Answer from the drawing. Dimensions are ordinates in mm from the lowest x, y and z of the part. Coordinates: 2 decimals unless noted, no trailing zeros. Loops run counter-clockwise (first coordinate to the right, second up) from the corner with the lowest first, then second, coordinate; pieces in that order, holes last. Notation, with made-up numbers: (7, -30.5) -> (65, -30.5) arc R24 cw to (65, -12.5) -> close; hole circle Ø10 at (-30.75, -9.75). An arc over 180 degrees is marked (long way). Use a Markdown table: item, result.
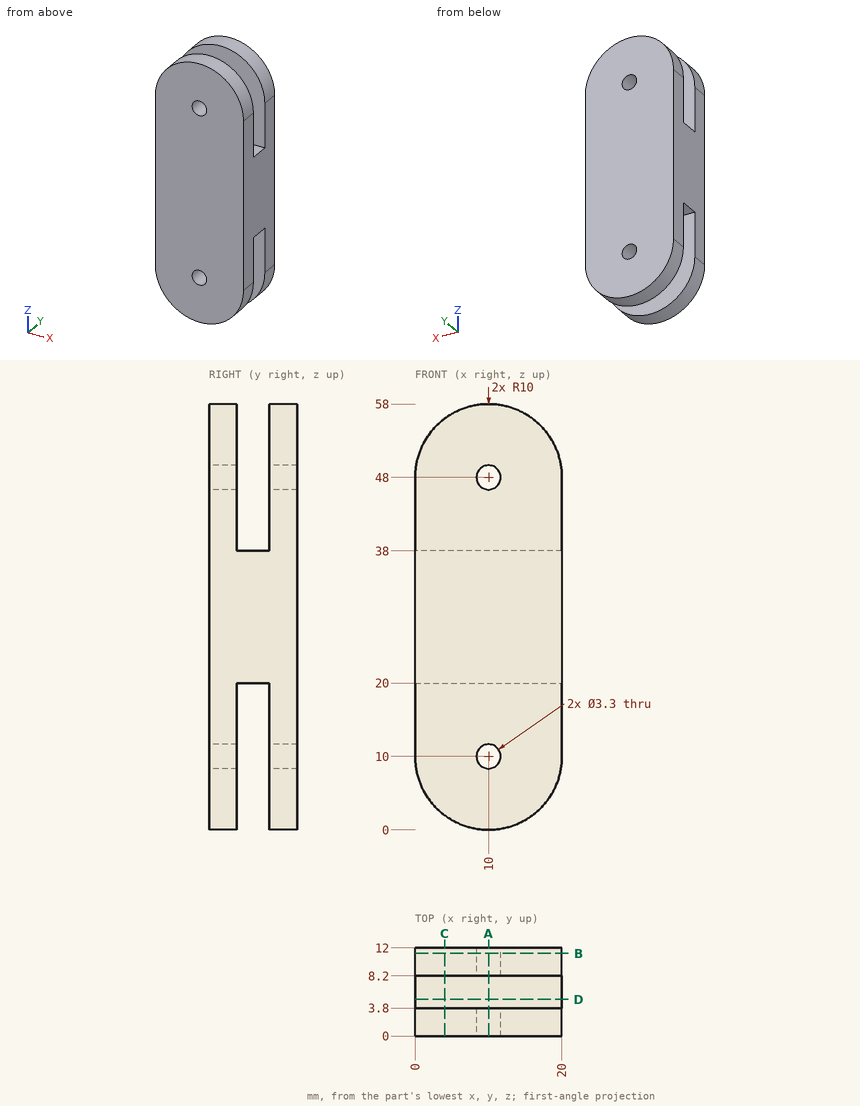
Q1. Consider line 1 (Z direction, x = 10, y = 10.1); line 2 (Y direction, x = 6, z = 8.5); line 3 (X direction, y = 9, z = 9). Determine where each line is inside the solid, lowest interval first. Write a range as [from, to].
Solved:
| item | result |
|---|---|
| line 1 | [0, 8.35], [11.65, 46.35], [49.65, 58] |
| line 2 | [0, 3.8], [8.2, 12] |
| line 3 | [0.05, 8.69], [11.31, 19.95] |
Q2. Section C-C on x = 4 is taken. Determine the outline of the cut face in (y, z).
Solved:
| item | result |
|---|---|
| outline | (0, 2) -> (3.8, 2) -> (3.8, 20) -> (8.2, 20) -> (8.2, 2) -> (12, 2) -> (12, 56) -> (8.2, 56) -> (8.2, 38) -> (3.8, 38) -> (3.8, 56) -> (0, 56) -> close |
Q3. Section B-B on y = 11.25 is taken. Determine the outline of the cut face in (x, z).
Solved:
| item | result |
|---|---|
| outline | (0, 10) arc R10 ccw to (20, 10) -> (20, 48) arc R10 ccw to (0, 48) -> close; hole circle Ø3.3 at (10, 10); hole circle Ø3.3 at (10, 48) |
Q4. Section A-A on x = 10 is taken. Determine the outline of the cut face in (y, z), and give its area (3 significant figures).
Solved:
| item | result |
|---|---|
| outline | (0, 0) -> (3.8, 0) -> (3.8, 8.35) -> (0, 8.35) -> close; (0, 11.65) -> (3.8, 11.65) -> (3.8, 20) -> (8.2, 20) -> (8.2, 11.65) -> (12, 11.65) -> (12, 46.35) -> (8.2, 46.35) -> (8.2, 38) -> (3.8, 38) -> (3.8, 46.35) -> (0, 46.35) -> close; (0, 49.65) -> (3.8, 49.65) -> (3.8, 58) -> (0, 58) -> close; (8.2, 0) -> (12, 0) -> (12, 8.35) -> (8.2, 8.35) -> close; (8.2, 49.65) -> (12, 49.65) -> (12, 58) -> (8.2, 58) -> close |
| area | 470 mm² |
Q5. Given pin 1 Ø3.5 at (x, y) = (10.5, 6) entering from +Z; pin 2 Ø5 at (x, y) = (13, 2.5) entering from +Z; pin 3 Ø2.5 at (x, z) = (10, 48) entering from +Y; pin 4 Ø2 at (x, y) = (12.5, 10) entering from +Z, each flat-ended and moving along its own axis, determine where each tip first touches the part or whether it passes through.
Solved:
| item | result |
|---|---|
| pin 1 | z = 38 |
| pin 2 | z = 57.99 |
| pin 3 | through |
| pin 4 | z = 57.89 |
Q6. Section D-D on y = 5 is taken. Determine the outline of the cut face in (x, z), and give its area (3 significant figures).
Solved:
| item | result |
|---|---|
| outline | (0, 20) -> (20, 20) -> (20, 38) -> (0, 38) -> close |
| area | 360 mm² |
